from build123d import *

# Parameters (mm, degrees)
SKETCH1_R                          = 7.9375
SKETCH1_R_2                        = 6.4375
PIPE_CONFIGURED_21_3_X_2_3_3_DEPTH = 415.043480752
CORTE_EXTRUS_O1_DEPTH              = 562.915780451
CORTE_EXTRUS_O1_DEPTH_BACK         = 562.915780451
ESBO_O10_R                         = 7.9375
CORTE_EXTRUS_O2_DEPTH              = 562.915780609
CORTE_EXTRUS_O2_DEPTH_BACK         = 562.915780609
ESBO_O11_R                         = 7.9375


with BuildPart() as part:
    # Sketch1 → Pipe - configured 21.3 X 2.3(3) (new body)
    with BuildSketch(Plane(origin=(58.531578249, 250, -150), x_dir=(0, 0, -1), z_dir=(1, 0, 0))):
        Circle(SKETCH1_R)
        Circle(SKETCH1_R_2, mode=Mode.SUBTRACT)
    extrude(amount=PIPE_CONFIGURED_21_3_X_2_3_3_DEPTH)

    # Esboço10 → Corte-extrusão1 (cut, two sides: drawn at the far end of the back side and taken through both)
    with BuildSketch(Plane.XY.offset(-CORTE_EXTRUS_O1_DEPTH_BACK)):
        with Locations((58.531578249, 250)):
            Circle(ESBO_O10_R)
    extrude(amount=CORTE_EXTRUS_O1_DEPTH + CORTE_EXTRUS_O1_DEPTH_BACK, mode=Mode.SUBTRACT)

    # Esboço11 → Corte-extrusão2 (cut, two sides: drawn at the far end of the back side and taken through both)
    with BuildSketch(Plane.XY.offset(-CORTE_EXTRUS_O2_DEPTH_BACK)):
        with Locations((473.575059, 250)):
            Circle(ESBO_O11_R)
    extrude(amount=CORTE_EXTRUS_O2_DEPTH + CORTE_EXTRUS_O2_DEPTH_BACK, mode=Mode.SUBTRACT)


solid = part.part
Here's how the part is built. I have some questions about the finished solid (model axes, mm). Coordinates: 2 decimals unless noted, no trailing zeros. Order: outer loops, then holes, each group sorted by start corner. A loop starts at its lowest first (then second) coordinate and runs counter-clockwise, first axis right, second up. Notation, with made-up numbers: (-15.75, -8) -> (30.25, -8) arc R23 ccw to (30.25, 19) -> close; hole circle Ø2 at (-36.5, 48). An arc over 180 degrees is marked (long way). Answer in a Markdown table with one row per item.
(1) I want a section at A-A on z = -150. List the corners of the cut face in (x, y) for me (1 decimal), then the cut area to 3 significant figures.
Answer key:
| item | result |
|---|---|
| outline | (58.5, 242.1) -> (473.6, 242.1) arc R7.9 cw to (468.9, 243.6) -> (63.2, 243.6) arc R7.9 cw to start; (58.5, 257.9) arc R7.9 cw to (63.2, 256.4) -> (468.9, 256.4) arc R7.9 cw to (473.6, 257.9) -> close |
| area | 1,230 mm^2 |
(2) Thinking about a two-plate mould opening in Y: for faces 1 (the face through (263.148, 242.958, -153.663)), 2 (the face through (263.21, 250.28, -143.57)), which applies, +Y half, -Y half, draft (parallel to the pull), parting line (faces both ways), or undercut?
Answer key:
| item | result |
|---|---|
| face 1 | parting line |
| face 2 | undercut |
(3) I want a section at B-B on y = 250. List the corners of the cut face in (x, z) for me, then the cut area to 3 significant figures.
Answer key:
| item | result |
|---|---|
| outline | (66.47, -157.94) -> (465.64, -157.94) -> (465.64, -156.44) -> (66.47, -156.44) -> close; (66.47, -143.56) -> (465.64, -143.56) -> (465.64, -142.06) -> (66.47, -142.06) -> close |
| area | 1,200 mm^2 |
(4) Will these pins go through, and if not, where does the flat tip stop? pin 1 Ø1 at (y, z) = (254.5, -150) entering from -X; pin 2 Ø6 at (y, z) = (256, -152.5) entering from -X; pin 3 Ø1 at (y, z) = (247.5, -156) entering from -X; pin 4 Ø1.5 at (x, y) = (357.5, 252) entering from -Z.
Answer key:
| item | result |
|---|---|
| pin 1 | through |
| pin 2 | x = 58.74 |
| pin 3 | x = 65.88 |
| pin 4 | z = -157.84 |
(5) I want a section at C-C on x = 343.5. List the corners of the cut face in (y, z) for me (1 decimal).
Answer key:
| item | result |
|---|---|
| outline | circle Ø15.9 at (250, -150); hole circle Ø12.9 at (250, -150) |
(6) Please list where these lines run through material, in increasing order: probe 1 along Z at (x, y) = (286, 250); probe 2 along Y at (x, z) = (166.5, -149); probe 3 along Y at (x, z) = (297.5, -145).
Answer key:
| item | result |
|---|---|
| probe 1 | -157.94 to -156.44, -143.56 to -142.06 |
| probe 2 | 242.13 to 243.64, 256.36 to 257.87 |
| probe 3 | 243.84 to 245.95, 254.05 to 256.16 |
